from build123d import *

# Parameters (mm, degrees)
SKETCH1_W           = 41.95
SKETCH1_H           = 31.993
BOSS_EXTRUDE1_DEPTH = 0.5
SKETCH2_W           = 1
SKETCH2_H           = 1
BOSS_EXTRUDE2_DEPTH = 10
LPATTERN1_COUNT     = 5
LPATTERN1_PITCH     = 10.23


with BuildPart() as part:
    # Sketch1 → Boss-Extrude1 (new, symmetric)
    with BuildSketch(Plane.XY):
        Rectangle(SKETCH1_W, SKETCH1_H)
        with BuildLine():
            Line((18.475, -14.4965), (-18.475, -14.4965))
            ThreePointArc((-18.475, -14.4965), (-20.182106781, -15.203606781), (-19.475, -13.4965))
            Line((-19.475, -13.4965), (-19.475, 14.4965))
            Line((-19.475, 14.4965), (19.475, 14.4965))
            Line((19.475, 14.4965), (19.475, -13.4965))
            ThreePointArc((19.475, -13.4965), (20.182106781, -13.789393219), (20.475, -14.4965))
            ThreePointArc((20.475, -14.4965), (19.475, -15.4965), (18.475, -14.4965))
        make_face(mode=Mode.SUBTRACT)
    extrude(amount=BOSS_EXTRUDE1_DEPTH, both=True)

    # Sketch2 → Boss-Extrude2 (add)
    with BuildSketch(Plane(origin=(0, 15.9965, 0), x_dir=(1, 0, 0), z_dir=(0, 1, 0))):
        with Locations((-20.475, 0)):
            Rectangle(SKETCH2_W, SKETCH2_H)
    boss_extrude2 = extrude(amount=BOSS_EXTRUDE2_DEPTH)

    # LPattern1: Boss-Extrude2 ×5
    with Locations(*[(i * LPATTERN1_PITCH, 0, 0) for i in range(1, LPATTERN1_COUNT)]):
        add(boss_extrude2)


solid = part.part
Verification items for the finished model (mm, model axes). A direction names the side the tool comes from. Round coordinates to 2 decimals unless told otherwise and drop trailing zeros. Loops run counter-clockwise (first coordinate to the right, second up) from the corner with the lowest first, then second, coordinate; pieces in that order, holes last. Notation, with made-up numbers: (27, -19.75) - (81, -19.75) arc R37 ccw to (81, 17.25) - close; hole circle Ø8 at (56, 24.25). An arc over 180 degrees is marked (long way). Write item = value, one per line.
Q1. Sectioned sample at B-B on x = -4. Record the boundary of the cut face in (y, z).
Here are the results:
outline = (-16, -0.5) - (-14.5, -0.5) - (-14.5, 0.5) - (-16, 0.5) - close; (14.5, -0.5) - (16, -0.5) - (16, 0.5) - (14.5, 0.5) - close
Q2. Sectioned sample at A-A on y = 7.5. Record the boundary of the cut face in (x, z) (3 decimals), plus the area to 3 significant figures.
Here are the results:
outline = (-20.975, -0.5) - (-19.475, -0.5) - (-19.475, 0.5) - (-20.975, 0.5) - close; (19.475, -0.5) - (20.975, -0.5) - (20.975, 0.5) - (19.475, 0.5) - close
area = 3.00 mm^2
Q3. Tool access check on faces 1 (the flat face through (0, -14.496, 0)), 2 (the flat face through (0, 25.996, 0)), 3 (the flat face through (0.485, 21, 0)). Record the directions out of +Z, -Z, +X, -X, +Y, -Y that give a thin tool (end or side, any length) a straight path to the whole face; none if there is none.
Here are the results:
face_1 = +Z, -Z
face_2 = +Z, -Z, +X, -X, +Y
face_3 = +Z, -Z, +Y
Q4. Depth check by flat-ended pin: pin 1 (0.5 mm diameter, centred on y = 22.5, z = 0, fed in from +X) (3 decimals). Enter the tip coordinate at first touch or a pass-through.
Here are the results:
pin_1 = 20.945
Q5. Sectioned sample at C-C on y = 18. Record the boundary of the cut face in (x, z) (3 decimals).
Here are the results:
outline = (-20.975, -0.5) - (-19.975, -0.5) - (-19.975, 0.5) - (-20.975, 0.5) - close; (-10.745, -0.5) - (-9.745, -0.5) - (-9.745, 0.5) - (-10.745, 0.5) - close; (-0.515, -0.5) - (0.485, -0.5) - (0.485, 0.5) - (-0.515, 0.5) - close; (9.715, -0.5) - (10.715, -0.5) - (10.715, 0.5) - (9.715, 0.5) - close; (19.945, -0.5) - (20.945, -0.5) - (20.945, 0.5) - (19.945, 0.5) - close
Q6. Mould release check, pull along Y, two halves, no side actions. Record for faces 4 (the flat face through (-10.745, 21, 0)), 5 (the cylindrical face through (20.205, -15.18, 0.007)), 6 (the flat face through (-20.5, 25.996, 0)): +Y half, -Y half, draft (parallel to the pull), parting line (faces both ways), or undercut.
Here are the results:
face_4 = draft
face_5 = undercut
face_6 = +Y half
Q7. Material ranges on L1, parallel to X at y = 18, z = -0.15 (3 decimals); L2, parallel to X at y = -13, z = -0.4 (3 decimals); L3, parallel to Y at x = -9, z = -0.25, recorded low to high.
Here are the results:
L1 = -20.975 to -19.975, -10.745 to -9.745, -0.515 to 0.485, 9.715 to 10.715, 19.945 to 20.945
L2 = -20.975 to -19.475, 19.475 to 20.975
L3 = -16 to -14.5, 14.5 to 16
